The listing builds one solid part. Answer for the finished solid, in the listing's coordinates (mm). A direction names the side the tool comes from. Round coordinates to 2 decimals unless told otherwise and drop trailing zeros. Order: outer loops, then holes, each group sorted by start corner. A loop starts at its lowest first (then second) coordinate and runs counter-clockwise, first axis right, second up. Notation, with made-up numbers: M -38,-26 L 17,-26 A24 ccw 17,-16 Z; hole C -25,74 d1. An arc over 180 degrees is marked long. Write item = value, one per line. Start each with the question number.
(1) Straight lines are drawn through the part: probe 1 along Y at (x, z) = (-35.85, 32.5); probe 2 along X at (y, z) = (5, 30). For each, find the intervals that lie inside material, in ascending order. Write a range as from..to.
(2) A cutting plane is placed at A-A, the plane z = 32.5. Determine the outline of the cut face in (x, y), and give its area (3 significant figures).
(3) Each of these flat-tipped pins is pushed along its axis until it touches: pin 1 (1.7 mm diameter, centred on y = 3, z = -39.5, fed in from -X); pin 2 (3.5 mm diameter, centred on y = 4, z = -40, fed in from +X). Where does it stop, or does it pass through?
(4) A cutting plane is placed at B-B, the plane y = 4. Determine the outline of the cut face in (x, z).
(5) Which of the six approach directions +Z, -Z, +X, -X, +Y, -Y give full straight-line access (tool end or side, diameter ignored) to faces 4 (the face through (37.5, 4, 1)), 5 (the face through (-32.6, 4, 33)), 6 (the face through (32.6, 4, -40))?
(6) For a pull along Y with two mould halves and no side action, classify faces 1 (the face through (32.6, 4, 33)), 2 (the face through (-1, 0, -1)), 3 (the face through (-1, 4, 45)) as released by +Y, released by -Y, zero draft, split by the parting line, or undercut.
from build123d import *

# Parameters (mm, degrees)
SKETCH1_W           = 75
SKETCH1_H           = 90
BOSS_EXTRUDE1_DEPTH = 8
SKETCH2_R           = 2.8
CUT_EXTRUDE1_DEPTH  = 4.9


with BuildPart() as part:
    # Sketch1 → Boss-Extrude1 (new body)
    with BuildSketch(Plane(origin=(0, 0, 0), x_dir=(1, 0, 0), z_dir=(0, 1, 0))):
        Rectangle(SKETCH1_W, SKETCH1_H)
    extrude(amount=BOSS_EXTRUDE1_DEPTH)

    # Sketch2 → Cut-Extrude1 (cut)
    with BuildSketch(Plane(origin=(37.5, 0, 0), x_dir=(0, 0, -1), z_dir=(1, 0, 0))):
        with Locations((40, 4)):
            Circle(SKETCH2_R)
        with Locations((-32.5, 4)):
            Circle(SKETCH2_R)
    cut_extrude1 = extrude(amount=-CUT_EXTRUDE1_DEPTH, mode=Mode.SUBTRACT)

    # Mirror1: Cut-Extrude1 across plane
    add(cut_extrude1.mirror(Plane(origin=(0, 0, 0), x_dir=(0, 0, 1), z_dir=(1, 0, 0))), mode=Mode.SUBTRACT)


solid = part.part
Reported:
q1.probe_1 = 0..1.2, 6.8..8
q1.probe_2 = -32.6..32.6
q2.outline = M -37.5,0 L 37.5,0 L 37.5,1.2 L 32.6,1.2 L 32.6,6.8 L 37.5,6.8 L 37.5,8 L -37.5,8 L -37.5,6.8 L -32.6,6.8 L -32.6,1.2 L -37.5,1.2 Z
q2.area = 545 mm²
q3.pin_1 = -32.6
q3.pin_2 = 32.6
q4.outline = M -37.5,-45 L 37.5,-45 L 37.5,-42.8 L 32.6,-42.8 L 32.6,-37.2 L 37.5,-37.2 L 37.5,29.7 L 32.6,29.7 L 32.6,35.3 L 37.5,35.3 L 37.5,45 L -37.5,45 L -37.5,35.3 L -32.6,35.3 L -32.6,29.7 L -37.5,29.7 L -37.5,-37.2 L -32.6,-37.2 L -32.6,-42.8 L -37.5,-42.8 Z
q5.face_4 = +Z, -Z, +X, +Y, -Y
q5.face_5 = -X
q5.face_6 = +X
q6.face_1 = undercut
q6.face_2 = released by -Y
q6.face_3 = zero draft
